Input: part model. Units: mm. Frame: model coordinates. A direction names the side the tool comes from. Round coordinates to 2 decimals unless told otherwise and drop trailing zeros. Loops run counter-clockwise (first coordinate to the right, second up) from the corner with the lowest first, then second, coordinate; pieces in that order, holes last. Notation, with made-up numbers: (-10, 5.25) -> (46, 5.25) arc R25 cw to (46, 19.25) -> close; hole circle Ø3 at (-5, 87.5). An arc over 180 degrees is marked (long way). One line per question, with ' | ' between items. Start each with the question number.
Q1. Cut plane A-A on x = 16. Return loops of the section in (y, z).
Q2. Mould query, pull axis Z, two halves, no side actions, for faces 1 (the face through (-14, -3, -4.1)), 2 (the face through (12, -3, 20)), 3 (the face through (-5, -230, 0)). Classes: pulls with the +Z half, pulls with the -Z half, needs draft (parallel to the pull), parting line crosses it, or undercut.
Q3. Contact query for flat-ended pins moving along their axis: P1, Ø2.5, axis at x = -0.5, y = 69, coming from the +Z side; P2, Ø4, axis at y = 2, z = 0.5, coming from the -X side; P3, Ø6.5, axis at x = 0.5, y = 18, coming from the -Z side. Output: stop coordinate, or through.
Q4. Material intervals for L1, parallel to Z at x = -15, y = -182.5; L2, parallel to X at y = 135, z = 0, sorted ascending.
Q5. Cut plane B-B on y = 178. Return loops of the section in (x, z), and give its area (3 significant figures).
Q6. Access query for faces 4 (the face through (0, -3, -8)), 5 (the face through (14, -3, -4.1)), 6 (the face through (0, -3, 8)), 7 (the face through (-14, -3, 4.1)). Directions: +Z, -Z, +X, -X, +Y, -Y. A direction counts if a zero-diameter tool reaches every point of the face in a straight line with its end or side. Return the directions, or none.
from build123d import *

# Parameters (mm, degrees)
AUFSATZ_LINEAR_AUSTRAGEN1_DEPTH      = 230
AUFSATZ_LINEAR_AUSTRAGEN1_DEPTH_BACK = 230
SKIZZE1_R                            = 3.5


with BuildPart() as part:
    # Skizze1 → Aufsatz-Linear austragen1 (new, two sides: drawn at the far end of the back side and taken through both)
    with BuildSketch(Plane(origin=(0, 0, 0), x_dir=(1, 0, 0), z_dir=(0, 1, 0)).offset(-AUFSATZ_LINEAR_AUSTRAGEN1_DEPTH_BACK)):
        Polygon((-4.1, -20), (-4.1, -8), (4.1, -8), (4.1, -20), (20, -20), (20, -4.1), (8, -4.1), (8, 4.1), (20, 4.1), (20, 20), (4.1, 20), (4.1, 8), (-4.1, 8), (-4.1, 20), (-20, 20), (-20, 4.1), (-8, 4.1), (-8, -4.1), (-20, -4.1), (-20, -20), align=None)
        with Locations(Location((0, 0, 0), (0, 0, 270))):
            Circle(SKIZZE1_R, mode=Mode.SUBTRACT)
    extrude(amount=AUFSATZ_LINEAR_AUSTRAGEN1_DEPTH + AUFSATZ_LINEAR_AUSTRAGEN1_DEPTH_BACK)


solid = part.part
Results:
1) outline: (-230, -20) -> (230, -20) -> (230, -4.1) -> (-230, -4.1) -> close; (-230, 4.1) -> (230, 4.1) -> (230, 20) -> (-230, 20) -> close
2) face 1: undercut | face 2: pulls with the +Z half | face 3: needs draft
3) P1: z = 8 | P2: x = -8 | P3: z = -8
4) L1: -20 to -4.1, 4.1 to 20 | L2: -8 to -3.5, 3.5 to 8
5) outline: (-20, -20) -> (-4.1, -20) -> (-4.1, -8) -> (4.1, -8) -> (4.1, -20) -> (20, -20) -> (20, -4.1) -> (8, -4.1) -> (8, 4.1) -> (20, 4.1) -> (20, 20) -> (4.1, 20) -> (4.1, 8) -> (-4.1, 8) -> (-4.1, 20) -> (-20, 20) -> (-20, 4.1) -> (-8, 4.1) -> (-8, -4.1) -> (-20, -4.1) -> close; hole circle Ø7 at (0, 0) | area: 1,170 mm^2
6) face 4: -Z, +Y, -Y | face 5: +X, +Y, -Y | face 6: +Z, +Y, -Y | face 7: -X, +Y, -Y
